Part model, mm, in its own coordinate system. Face numbers are marked on the shaded views. A direction names the side the tool comes from. Coordinates: 2 decimals unless noted, no trailing zeros. Write each loop counter-clockwise with the first axis right and the second up, starting at its lowest first coordinate (ties: lowest second). Pieces come first, ordered by that corner, then holes. Notation, with made-up numbers: (-38, -5.75) -> (14, -5.75) arc R25 cw to (14, 24.25) -> close; hole circle Ø3 at (88, -15.75). An arc over 180 degrees is marked (long way). Write item = value, one per line.
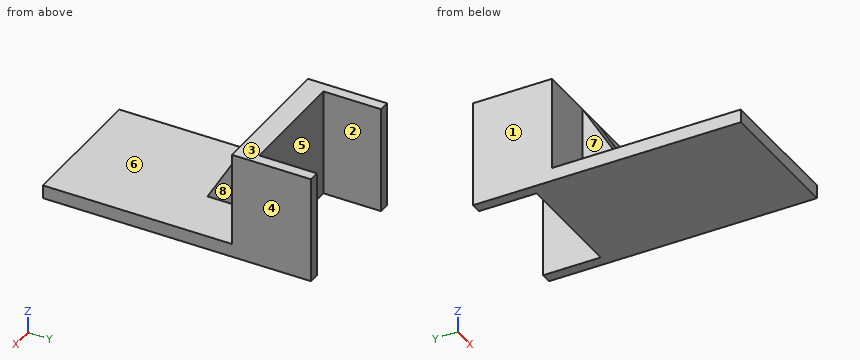
from build123d import *

# Parameters (mm, degrees)
EXTRUDE_1_DEPTH     = 5
EXTRUDE_2_DEPTH     = 5
CUT_EXTRUDE_2_DEPTH = 52
SKETCH_6_W          = 43
SKETCH_6_H          = 8
EXTRUDE_3_DEPTH     = 35
RIB_4_REACH         = 262.096
SKETCH_8_WALL_W     = 562.75395357
SKETCH_8_WALL_H     = 10
CUT_EXTRUDE_3_DEPTH = 35
SKETCH_10_W         = 141.906690428
SKETCH_10_H         = 100
CUT_EXTRUDE_4_DEPTH = 10


with BuildPart() as part:
    # 草图1 → 凸台-拉伸1 (new body)
    with BuildSketch(Plane.XY):
        with BuildLine():
            Line((167.406690428, -100), (0, -100))
            Line((0, -100), (-167.406690428, -100))
            ThreePointArc((-167.406690428, -100), (0, -195), (167.406690428, -100))
        make_face()
    extrude(amount=EXTRUDE_1_DEPTH)

    # 草图4 → 凸台-拉伸2 (add)
    with BuildSketch(Plane.XY.offset(5)):
        Polygon((167.406690428, 0), (0, 0), (0, -100), (21.5, -100), (167.406690428, -100), align=None)
        Polygon((0, -100), (0, 0), (-167.406690428, 0), (-167.406690428, -100), (-21.5, -100), align=None)
    extrude(amount=-EXTRUDE_2_DEPTH)

    # 草图5 → 切除-拉伸2 (cut)
    with BuildSketch(Plane.XY.offset(5)):
        Polygon((0, 0), (21.5, 0), (21.5, -21.5), (-21.5, -21.5), (-21.5, 0), align=None)
    extrude(amount=-CUT_EXTRUDE_2_DEPTH, mode=Mode.SUBTRACT)

    # 草图6 → 凸台-拉伸3 (add)
    with BuildSketch(Plane.XY.offset(5)):
        Polygon((-21.5, -29.5), (-21.5, -21.5), (-21.5, 0), (-25.5, 0), (-25.5, -29.5), align=None)
        with Locations((0, -25.5)):
            Rectangle(SKETCH_6_W, SKETCH_6_H)
        Polygon((21.5, 0), (21.5, -21.5), (21.5, -29.5), (25.5, -29.5), (25.5, 0), align=None)
    extrude(amount=EXTRUDE_3_DEPTH)

    # 草图8 wall → 筋4 (add, up to next)
    with BuildSketch(Plane(origin=(0, -39.75, 22.5), x_dir=(0, -0.505403111507, -0.862883361109), z_dir=(0, 0.862883361109, -0.505403111507)), mode=Mode.PRIVATE) as rib_4_sk1:
        Rectangle(SKETCH_8_WALL_W, SKETCH_8_WALL_H)
    rib_4_tool1 = extrude(rib_4_sk1.sketch, amount=RIB_4_REACH, mode=Mode.PRIVATE) - part.part
    add(rib_4_tool1.solids().sort_by_distance((0, -39.75, 22.5))[0])

    # 草图9 → 切除-拉伸3 (cut)
    with BuildSketch(Plane(origin=(0, 0, 0), x_dir=(-1, 0, 0), z_dir=(0, 0, -1))):
        Polygon((-167.406690428, -100), (167.406690428, -100), (167.406690428, -206.368717501), (-177.688477613, -206.368717501), align=None)
    extrude(amount=-CUT_EXTRUDE_3_DEPTH, mode=Mode.SUBTRACT)

    # 草图10 → 切除-拉伸4 (cut)
    with BuildSketch(Plane(origin=(0, 0, 0), x_dir=(-1, 0, 0), z_dir=(0, 0, -1))):
        with Locations((-96.453345214, -50)):
            Rectangle(SKETCH_10_W, SKETCH_10_H)
        with Locations((96.453345214, -50)):
            Rectangle(SKETCH_10_W, SKETCH_10_H)
    extrude(amount=-CUT_EXTRUDE_4_DEPTH, mode=Mode.SUBTRACT)


solid = part.part
Q1. Saw through at D-D on y = -40.5. Give the cut face in (x, z), and give its area (3 significant figures).
Model answer:
outline = (-25.5, 0) -> (25.5, 0) -> (25.5, 5) -> (5, 5) -> (5, 21.22) -> (-5, 21.22) -> (-5, 5) -> (-25.5, 5) -> close
area = 417 mm²
Q2. Saw through at C-C on x = -12. Give the cut face in (y, z).
Model answer:
outline = (-100, 0) -> (-21.5, 0) -> (-21.5, 40) -> (-29.5, 40) -> (-29.5, 5) -> (-100, 5) -> close
Q3. Saw through at B-B on z = 8.5. Give the cut face in (x, y), and give its area (4 significant figures).
Model answer:
outline = (-25.5, -29.5) -> (-5, -29.5) -> (-5, -47.95) -> (5, -47.95) -> (5, -29.5) -> (25.5, -29.5) -> (25.5, 0) -> (21.5, 0) -> (21.5, -21.5) -> (-21.5, -21.5) -> (-21.5, 0) -> (-25.5, 0) -> close
area = 764.5 mm²
Q4. Probe line 1 (X direction, y = -36, z = 26.5); line 2 (Z direction, x = 9, y = -57); line 3 (Y direction, x = 17.5, z = 8.5). List the from-to ranges inside material, lowest first. Write a range as from..to.
Model answer:
line_1 = -5..5
line_2 = 0..5
line_3 = -29.5..-21.5
Q5. Pin check, flat tips, straight feed: pin 1 (16.5 mm diameter, centred on x = -14.5, z = 27.5, fed in from -Y); pin 2 (6 mm diameter, centred on y = -43.5, z = 21, fed in from +X); pin 3 (5 mm diameter, centred on x = 13.5, z = 31.5, fed in from +Y); pin 4 (10.5 mm diameter, centred on y = -42.5, z = 29, fed in from -X). Stop position of each tip, or through.
Model answer:
pin_1 = -29.5
pin_2 = 5
pin_3 = -21.5
pin_4 = through
Q6. Mould opens along X. For the marked faces 1, 2 and 3 say: released by +X, released by -X, zero draft, split by the parting line, or undercut.
Model answer:
face_1 = released by -X
face_2 = undercut
face_3 = zero draft
Q7. Which spindle directions (+Z, -Z, +X, -X, +Y, -Y) get a long thin tool onto all of the face, cutting with end or side? Do the marked faces 4, 5, 6, 7 and 8. Say none if no direction does.
Model answer:
face_4 = +Z, -Z, +X, +Y, -Y
face_5 = +Z, -Z, +Y
face_6 = +Z, -Y
face_7 = +Z, -X, -Y
face_8 = +Z, +X, -Y
Q8. Saw through at A-A on y = -20. Give the cut face in (x, z).
Model answer:
outline = (-25.5, 0) -> (-21.5, 0) -> (-21.5, 40) -> (-25.5, 40) -> close; (21.5, 0) -> (25.5, 0) -> (25.5, 40) -> (21.5, 40) -> close
